from build123d import *

# Parameters (mm, degrees)
SKETCH1_W                = 108.6
SKETCH1_H                = 95.4
BOSS_EXTRUDE1_DEPTH      = 16.1
CUT_EXTRUDE1_DEPTH       = 75.047214667
FILLET1_R                = 4.7
SHELL1_T                 = -3
SHELL1_THICKNESS_2_DEPTH = 1
CUT_EXTRUDE2_DEPTH       = 1.5
SKETCH4_W                = 78.8
SKETCH4_H                = 51.8
CUT_EXTRUDE3_DEPTH       = 74.63823735
SKETCH5_W                = 82.6
SKETCH5_H                = 55.6
SKETCH5_W_2              = 78.8
SKETCH5_H_2              = 51.8
BOSS_EXTRUDE2_DEPTH      = 3
SKETCH6_R                = 4
SKETCH6_R_2              = 1
CUT_EXTRUDE4_DEPTH       = 74.63823735
BOSS_EXTRUDE3_START      = 2.8
BOSS_EXTRUDE3_DEPTH      = 2.8
CHAMFER1_SIZE            = 1.5
CUT_EXTRUDE5_REACH       = 121.702
SKETCH8_W                = 2.9
SKETCH8_H                = 30
BOSS_EXTRUDE4_START      = 8
BOSS_EXTRUDE4_DEPTH      = 8
FILLET2_R                = 2.9
SKETCH10_R               = 1.21
CUT_EXTRUDE6_DEPTH       = 9


with BuildPart() as part:
    # Sketch1 → Boss-Extrude1 (new body)
    with BuildSketch(Plane.XY):
        Rectangle(SKETCH1_W, SKETCH1_H)
    extrude(amount=BOSS_EXTRUDE1_DEPTH)

    # Sketch2 → Cut-Extrude1 (cut, through all)
    with BuildSketch(Plane.XY.offset(16.1)):
        with BuildLine():
            Line((50.011, -6.861266451), (50.011, 21.582126451))
            ThreePointArc((50.011, 21.582126451), (148.66075, 7.36043), (50.011, -6.861266451))
        make_face()
    extrude(amount=-CUT_EXTRUDE1_DEPTH, mode=Mode.SUBTRACT)

    # Fillet1
    fillet1_edges = [part.edges().sort_by_distance(p)[0] for p in [
        (54.3, -47.7, 8.05),
        (-54.3, -47.7, 8.05),
        (-54.3, 47.7, 8.05),
        (54.3, 47.7, 8.05),
    ]]
    fillet(fillet1_edges, radius=FILLET1_R)

    # Shell1
    shell1_openings = [part.faces().sort_by_distance(p)[0] for p in [
        (-0.877010034, -0.123339484, 16.1),
    ]]
    offset(amount=SHELL1_T, openings=shell1_openings, kind=Kind.INTERSECTION)

    # Shell1 thickness 2 face (on inner face of the shell) → Shell1 thickness 2 (cut)
    with BuildSketch(Plane(origin=(-0.963593996, -0.143755332, 3), x_dir=(-1, 0, 0), z_dir=(0, 0, -1))):
        with BuildLine():
            Line((50.336406004, 43.143755332), (50.336406004, -42.856244668))
            ThreePointArc((50.336406004, -42.856244668), (49.838487532, -44.058326196), (48.636406004, -44.556244668))
            Line((48.636406004, -44.556244668), (-50.563593996, -44.556244668))
            ThreePointArc((-50.563593996, -44.556244668), (-51.765675524, -44.058326196), (-52.263593996, -42.856244668))
            Line((-52.263593996, -42.856244668), (-52.263593996, -17.719055626))
            ThreePointArc((-52.263593996, -17.719055626), (-49.835507324, -12.546349038), (-47.974593996, -7.143618255))
            Line((-47.974593996, -7.143618255), (-47.974593996, 22.151988919))
            ThreePointArc((-47.974593996, 22.151988919), (-49.835507324, 27.554719702), (-52.263593996, 32.72742629))
            Line((-52.263593996, 32.72742629), (-52.263593996, 43.143755332))
            ThreePointArc((-52.263593996, 43.143755332), (-51.765675524, 44.34583686), (-50.563593996, 44.843755332))
            Line((-50.563593996, 44.843755332), (48.636406004, 44.843755332))
            ThreePointArc((48.636406004, 44.843755332), (49.838487532, 44.34583686), (50.336406004, 43.143755332))
        make_face()
    extrude(amount=SHELL1_THICKNESS_2_DEPTH, mode=Mode.SUBTRACT)

    # Sketch3 → Cut-Extrude2 (cut)
    with BuildSketch(Plane.XY.offset(16.1)):
        with BuildLine():
            Line((-51.3, 43), (-51.3, -43))
            ThreePointArc((-51.3, -43), (-50.802081528, -44.202081528), (-49.6, -44.7))
            Line((-49.6, -44.7), (49.6, -44.7))
            ThreePointArc((49.6, -44.7), (50.802081528, -44.202081528), (51.3, -43))
            Line((51.3, -43), (51.3, -17.862810958))
            ThreePointArc((51.3, -17.862810958), (48.786619627, -12.478496653), (46.887595336, -6.84807676))
            Line((46.887595336, -6.84807676), (48.549511715, -6.84807676))
            ThreePointArc((48.549511715, -6.84807676), (50.429997664, -12.273623472), (52.9, -17.457432205))
            Line((52.9, -17.457432205), (52.9, -43))
            ThreePointArc((52.9, -43), (51.933452378, -45.333452378), (49.6, -46.3))
            Line((49.6, -46.3), (-49.6, -46.3))
            ThreePointArc((-49.6, -46.3), (-51.933452378, -45.333452378), (-52.9, -43))
            Line((-52.9, -43), (-52.9, 43))
            ThreePointArc((-52.9, 43), (-51.933452378, 45.333452378), (-49.6, 46.3))
            Line((-49.6, 46.3), (49.6, 46.3))
            ThreePointArc((49.6, 46.3), (51.933452378, 45.333452378), (52.9, 43))
            Line((52.9, 43), (52.9, 32.178292205))
            ThreePointArc((52.9, 32.178292205), (50.429997664, 26.994483472), (48.549511715, 21.56893676))
            Line((48.549511715, 21.56893676), (46.887595336, 21.56893676))
            ThreePointArc((46.887595336, 21.56893676), (48.786619627, 27.199356653), (51.3, 32.583670958))
            Line((51.3, 32.583670958), (51.3, 43))
            ThreePointArc((51.3, 43), (50.802081528, 44.202081528), (49.6, 44.7))
            Line((49.6, 44.7), (-49.6, 44.7))
            ThreePointArc((-49.6, 44.7), (-50.802081528, 44.202081528), (-51.3, 43))
        make_face()
    extrude(amount=-CUT_EXTRUDE2_DEPTH, mode=Mode.SUBTRACT)

    # Sketch4 → Cut-Extrude3 (cut, through all)
    with BuildSketch(Plane.XY.offset(2)):
        with Locations((0, 7.8)):
            Rectangle(SKETCH4_W, SKETCH4_H)
    extrude(amount=-CUT_EXTRUDE3_DEPTH, mode=Mode.SUBTRACT)

    # Sketch5 → Boss-Extrude2 (add)
    with BuildSketch(Plane.XY.offset(2)):
        with Locations((0, 7.8)):
            Rectangle(SKETCH5_W, SKETCH5_H)
        with Locations((0, 7.8)):
            Rectangle(SKETCH5_W_2, SKETCH5_H_2, mode=Mode.SUBTRACT)
    extrude(amount=BOSS_EXTRUDE2_DEPTH)

    # Sketch6 → Cut-Extrude4 (cut, through all)
    with BuildSketch(Plane.XY.offset(2)):
        with Locations((-36.35, -35.4)):
            Circle(SKETCH6_R)
        with Locations((-19.08998, -32.69324)):
            Circle(SKETCH6_R_2)
        with Locations((-19.08998, -37.3744)):
            Circle(SKETCH6_R_2)
        with Locations((-21.43056, -35.03382)):
            Circle(SKETCH6_R_2)
        with Locations((-16.7494, -35.03382)):
            Circle(SKETCH6_R_2)
        with BuildLine():
            Line((-0.7, -32.46283), (-0.7, -37.6))
            ThreePointArc((-0.7, -37.6), (-3.6, -40.5), (-6.5, -37.6))
            Line((-6.5, -37.6), (-6.5, -32.46283))
            ThreePointArc((-6.5, -32.46283), (-3.6, -29.56283), (-0.7, -32.46283))
        make_face()
    extrude(amount=-CUT_EXTRUDE4_DEPTH, mode=Mode.SUBTRACT)

    # Sketch7 → Boss-Extrude3 (add)
    with BuildSketch(Plane.XY.offset(2).offset(BOSS_EXTRUDE3_START)):
        with BuildLine():
            Line((-8.5, -32.46283), (-8.5, -37.6))
            ThreePointArc((-8.5, -37.6), (-3.6, -42.5), (1.3, -37.6))
            Line((1.3, -37.6), (1.3, -32.46283))
            ThreePointArc((1.3, -32.46283), (-3.6, -27.56283), (-8.5, -32.46283))
        make_face()
        with BuildLine():
            Line((-6.5, -32.46283), (-6.5, -37.6))
            ThreePointArc((-6.5, -37.6), (-3.6, -40.5), (-0.7, -37.6))
            Line((-0.7, -37.6), (-0.7, -32.46283))
            ThreePointArc((-0.7, -32.46283), (-3.6, -29.56283), (-6.5, -32.46283))
        make_face(mode=Mode.SUBTRACT)
    extrude(amount=-BOSS_EXTRUDE3_DEPTH)

    # Chamfer1
    chamfer1_edges = [part.edges().sort_by_distance(p)[0] for p in [
        (-3.6, -29.56283, 0),
        (-0.7, -35.031415, 0),
        (-3.6, -40.5, 0),
        (-6.5, -35.031415, 0),
    ]]
    chamfer(chamfer1_edges, length=CHAMFER1_SIZE)

    # Sketch8 → Cut-Extrude5 (cut, up to next)
    with BuildSketch(Plane(origin=(54.3, 0, 0), x_dir=(0, 0, -1), z_dir=(1, 0, 0)), mode=Mode.PRIVATE) as cut_extrude5_sk1:
        with Locations((-14.65, 7.36043)):
            Rectangle(SKETCH8_W, SKETCH8_H)
    cut_extrude5_tool1 = extrude(cut_extrude5_sk1.sketch, amount=-CUT_EXTRUDE5_REACH, mode=Mode.PRIVATE) & part.part
    add(cut_extrude5_tool1.solids().sort_by_distance((54.3, 7.36043, 14.65))[0], mode=Mode.SUBTRACT)

    # Sketch9 → Boss-Extrude4 (add)
    with BuildSketch(Plane.XY.offset(2).offset(BOSS_EXTRUDE4_START)):
        with BuildLine():
            Line((49.6, 44.7), (46.9, 44.7))
            Line((46.9, 44.7), (46.9, 40.1))
            Line((46.9, 40.1), (51.3, 40.1))
            Line((51.3, 40.1), (51.3, 43))
            ThreePointArc((51.3, 43), (50.802081528, 44.202081528), (49.6, 44.7))
        make_face()
        with BuildLine():
            Line((-51.3, 40.1), (-46.9, 40.1))
            Line((-46.9, 40.1), (-46.9, 44.7))
            Line((-46.9, 44.7), (-49.6, 44.7))
            ThreePointArc((-49.6, 44.7), (-50.802081528, 44.202081528), (-51.3, 43))
            Line((-51.3, 43), (-51.3, 40.1))
        make_face()
        with BuildLine():
            Line((-51.3, -43), (-51.3, -40.1))
            Line((-51.3, -40.1), (-46.9, -40.1))
            Line((-46.9, -40.1), (-46.9, -44.7))
            Line((-46.9, -44.7), (-49.6, -44.7))
            ThreePointArc((-49.6, -44.7), (-50.802081528, -44.202081528), (-51.3, -43))
        make_face()
        with BuildLine():
            Line((49.6, -44.7), (46.9, -44.7))
            Line((46.9, -44.7), (46.9, -40.1))
            Line((46.9, -40.1), (51.3, -40.1))
            Line((51.3, -40.1), (51.3, -43))
            ThreePointArc((51.3, -43), (50.802081528, -44.202081528), (49.6, -44.7))
        make_face()
    extrude(amount=-BOSS_EXTRUDE4_DEPTH)

    # Fillet2
    fillet2_edges = [part.edges().sort_by_distance(p)[0] for p in [
        (-46.9, 40.1, 6),
        (46.9, 40.1, 6),
        (46.9, -40.1, 6),
        (-46.9, -40.1, 6),
    ]]
    fillet(fillet2_edges, radius=FILLET2_R)

    # Sketch10 → Cut-Extrude6 (cut)
    with BuildSketch(Plane.XY.offset(10)):
        with Locations((-49.6, 43)):
            Circle(SKETCH10_R)
        with Locations((49.6, 43)):
            Circle(SKETCH10_R)
        with Locations((49.6, -43)):
            Circle(SKETCH10_R)
        with Locations((-49.6, -43)):
            Circle(SKETCH10_R)
    extrude(amount=-CUT_EXTRUDE6_DEPTH, mode=Mode.SUBTRACT)


solid = part.part
Input: part model. Units: mm. Frame: model coordinates. A direction names the side the tool comes from. Give positions to 0.01 mm unless a question says otherwise; leave off trailing zeros. Write each loop counter-clockwise with the first axis right and the second up, starting at its lowest first coordinate (ties: lowest second). Pieces come first, ordered by that corner, then holes.
Q1. Set-up query: faces 4 (the face through (48, 7, 13.2)), 5 (the face through (52.887, -46.36, 8.163)), 6 (the face through (1.3, -35, 3)), 7 (the face through (-3.531, -29.324, 1.26)), 8 (the face through (-0.7, -35, 3)). Return all of +Z, -Z, +X, -X, +Y, -Y with unobstructed straight access to the full face (end or side cutting, diameter ignored); none if empty.
Q2. Section D-D, the plane y = -25. Output: boundary loops of the cut face in (x, z).
Q3. Pull-direction query (X, two-part tool) for faces 1 (the face through (51.843, 26.747, 8.163)), 2 (the face through (49, 22.36, 14)), 3 (the face through (-1, -18.1, 2)); classes: pulls with the +X half, pulls with the -X half, needs draft (parallel to the pull), parting line crosses it, or undercut.
Q4. Material intervals for probe 1 along Y at (x, z) = (-38.5, 3); probe 2 along X at (y, z) = (-19, 13.25); probe 3 along Y at (x, z) = (-36.35, 0.9), sorted ascending.
Q5. Section C-C, the plane x = -36.35. Output: boundary loops of the cut face in (y, z).
Q6. First-contact query: P1, Ø2, axis at x = -49, y = -43, coming from the +Z side; P2, Ø2, axis at y = 1.5, z = 11.5, coming from the +X side; P3, Ø0.7, axis at x = 49.5, y = -42.5, coming from the +Z side. Flat tips, straight axial feed; report the tip coordinate or a pass-through.
Q7. Section A-A, the plane x = 18. Output: boundary loops of the cut face in (y, z), plus the area to 3 significant figures.
Q8. Section B-B, the plane y = 18. Output: boundary loops of the cut face in (x, z), plus the area to 3 significant figures.
Filled in:
1. face 4: +Z, +X
1. face 5: +Z, -Z, +X, -Y
1. face 6: +Z
1. face 7: -Z
1. face 8: +Z, -Z
2. outline: (-54.3, 0) - (54.3, 0) - (54.3, 16.1) - (52.9, 16.1) - (52.9, 14.6) - (51.3, 14.6) - (51.3, 2) - (-51.3, 2) - (-51.3, 14.6) - (-52.9, 14.6) - (-52.9, 16.1) - (-54.3, 16.1) - close
3. face 1: pulls with the +X half
3. face 2: needs draft
3. face 3: undercut
4. probe 1: y = -47.7 to -44.7, -20 to -18.1, 33.7 to 35.6, 44.7 to 47.7
4. probe 2: x = -54.3 to -51.3, 51.3 to 54.3
4. probe 3: y = -47.7 to -39.4, -31.4 to -18.1, 33.7 to 47.7
5. outline: (-47.7, 0) - (-39.4, 0) - (-39.4, 2) - (-44.7, 2) - (-44.7, 14.6) - (-46.3, 14.6) - (-46.3, 16.1) - (-47.7, 16.1) - close; (-31.4, 0) - (-18.1, 0) - (-18.1, 5) - (-20, 5) - (-20, 2) - (-31.4, 2) - close; (33.7, 0) - (47.7, 0) - (47.7, 16.1) - (46.3, 16.1) - (46.3, 14.6) - (44.7, 14.6) - (44.7, 2) - (35.6, 2) - (35.6, 5) - (33.7, 5) - close
6. P1: stops at z = 10
6. P2: stops at x = 50.01
6. P3: stops at z = 1
7. outline: (-47.7, 0) - (-18.1, 0) - (-18.1, 5) - (-20, 5) - (-20, 2) - (-44.7, 2) - (-44.7, 14.6) - (-46.3, 14.6) - (-46.3, 16.1) - (-47.7, 16.1) - close; (33.7, 0) - (47.7, 0) - (47.7, 16.1) - (46.3, 16.1) - (46.3, 14.6) - (44.7, 14.6) - (44.7, 2) - (35.6, 2) - (35.6, 5) - (33.7, 5) - close
7. area: 178 mm2
8. outline: (-54.3, 0) - (-39.4, 0) - (-39.4, 5) - (-41.3, 5) - (-41.3, 2) - (-51.3, 2) - (-51.3, 14.6) - (-52.9, 14.6) - (-52.9, 16.1) - (-54.3, 16.1) - close; (39.4, 0) - (50.01, 0) - (50.01, 13.2) - (47.01, 13.2) - (47.01, 2) - (41.3, 2) - (41.3, 5) - (39.4, 5) - close
8. area: 136 mm2
